The model under review builds one solid part; all positions refer to its coordinate system, in mm. A direction names the side the tool comes from. Coordinates: 2 decimals unless noted, no trailing zeros. Write each loop counter-clockwise with the first axis right and the second up, starting at its lowest first coordinate (ties: lowest second). Pieces come first, ordered by that corner, then holes.
1) For P1, Ø1.5, axis at y = -3.5, z = -2, coming from the -X side; P2, Ø1, axis at x = -19, y = -7, coming from the -Z side; P3, Ø3, axis at x = -7.5, z = -5, coming from the -Y side, all flat-tipped, find the tip position at first contact; note any pin that passes through.
2) Add section A-A, the plane x = -12.5. State the section outline as (y, z) points, then the cut area to 3 significant figures.
3) Add section B-B, the plane y = 0. State the section outline as (x, z) points, then the cut area to 3 significant figures.
4) Add section D-D, the plane z = -5.5. State the section outline as (x, y) points, then the cut area to 3 significant figures.
5) Machinability: for faces 4 (the flat face through (13.15, 2, -7)), 5 (the flat face through (0, -9.15, -7)), 6 (the flat face through (-17, 0, 3.8)), 7 (the flat face through (14.9, 0, 5)), which of the approach directions +Z, -Z, +X, -X, +Y, -Y give a long, thin tool a straight path to every point of the face, cutting with its end or side? Answer none if there is none.
6) Mouldability with a two-part tool opening along X and no side actions: class faces 1 (the flat face through (17, 0, 3.8)), 2 (the cylindrical face through (-18.4, 1.2, 1.9)), 3 (the cylindrical face through (23.727, 0.043, 1.927)) as released by +X, released by -X, zero draft, split by the parting line, or undercut.
7) For line 1 (X direction, y = -1.25, z = -1.5); line 2 (Z direction, x = -14.5, y = -5); line 3 (Y direction, x = 5.5, z = -5), list the stretches that pass through material, from the lowest coordinate up.
8) Add section C-C, the plane z = 0.75. State the section outline as (x, y) points, then the cut area to 3 significant figures.
from build123d import *

# Parameters (mm, degrees)
SKETCH1_W           = 29.8
SKETCH1_H           = 21.7
BOSS_EXTRUDE1_DEPTH = 5.4
SKETCH2_R           = 2
BOSS_EXTRUDE2_DEPTH = 3.8
FILLET1_R           = 4
BOSS_EXTRUDE3_DEPTH = 14.2


with BuildPart() as part:
    # Sketch1 → Boss-Extrude1 (new body)
    with BuildSketch(Plane.XY):
        Rectangle(SKETCH1_W, SKETCH1_H)
    extrude(amount=BOSS_EXTRUDE1_DEPTH)

    # Sketch2 → Boss-Extrude2 (add)
    # profile 1 of 2: a face of its own
    with BuildSketch(Plane.XY):
        Polygon((14.9, 10.85), (14.9, -10.85), (25.257485216, 0), align=None)
        with Locations(Location((20, 0, 0), (0, 0, 180))):
            Circle(SKETCH2_R, mode=Mode.SUBTRACT)
    # profile 2 of 2: a face of its own
    with BuildSketch(Plane.XY):
        Polygon((-14.9, 10.85), (-14.9, -10.85), (-25.257485216, 0), align=None)
        with Locations(Location((-20, 0, 0), (0, 0, 180))):
            Circle(SKETCH2_R, mode=Mode.SUBTRACT)
    extrude(amount=BOSS_EXTRUDE2_DEPTH)

    # Fillet1
    fillet1_edges = [part.edges().sort_by_distance(p)[0] for p in [
        (25.257485216, 0, 1.9),
        (-25.257485216, 0, 1.9),
    ]]
    fillet(fillet1_edges, radius=FILLET1_R)

    # Sketch3 → Boss-Extrude3 (add)
    with BuildSketch(Plane(origin=(0, 0, 0), x_dir=(-1, 0, 0), z_dir=(0, 0, -1))):
        Polygon((-13.15, 9.15), (13.15, 9.15), (13.15, -4), (8, -9.15), (-8, -9.15), (-13.15, -4), align=None)
    extrude(amount=BOSS_EXTRUDE3_DEPTH)


solid = part.part
Geometry results:
1. P1: stops at x = -13.15
1. P2: stops at z = 0
1. P3: stops at y = -9.15
2. outline: (-10.85, 0) - (-4.65, 0) - (-4.65, -14.2) - (9.15, -14.2) - (9.15, 0) - (10.85, 0) - (10.85, 5.4) - (-10.85, 5.4) - close
2. area: 313 mm2
3. outline: (-23.73, 0) - (-22, 0) - (-22, 3.8) - (-23.73, 3.8) - close; (-18, 0) - (-13.15, 0) - (-13.15, -14.2) - (13.15, -14.2) - (13.15, 0) - (18, 0) - (18, 3.8) - (14.9, 3.8) - (14.9, 5.4) - (-14.9, 5.4) - (-14.9, 3.8) - (-18, 3.8) - close; (22, 0) - (23.73, 0) - (23.73, 3.8) - (22, 3.8) - close
3. area: 571 mm2
4. outline: (-13.15, -4) - (-8, -9.15) - (8, -9.15) - (13.15, -4) - (13.15, 9.15) - (-13.15, 9.15) - close
4. area: 455 mm2
5. face 4: -Z, +X, +Y, -Y
5. face 5: -Z, +X, -X, -Y
5. face 6: +Z, -X, +Y, -Y
5. face 7: +Z, +X, +Y, -Y
6. face 1: zero draft
6. face 2: undercut
6. face 3: released by +X
7. line 1: x = -13.15 to 13.15
7. line 2: z = 0 to 5.4
7. line 3: y = -9.15 to 9.15
8. outline: (-22.62, -2.76) - (-14.9, -10.85) - (14.9, -10.85) - (22.62, -2.76) arc R4 ccw to (22.62, 2.76) - (14.9, 10.85) - (-14.9, 10.85) - (-22.62, 2.76) arc R4 ccw to start; hole circle Ø4 at (-20, 0); hole circle Ø4 at (20, 0)
8. area: 840 mm2
